from build123d import *

# Parameters (mm, degrees)
SKETCH1_W           = 44.45
SKETCH1_H           = 44.45
BOSS_EXTRUDE1_DEPTH = 6.35
SKETCH2_W           = 31.75
SKETCH2_H           = 31.75
BOSS_EXTRUDE2_DEPTH = 25.4
SKETCH3_W           = 44.45
SKETCH3_H           = 44.45
BOSS_EXTRUDE3_DEPTH = 6.35
SKETCH4_W           = 25.4
SKETCH4_H           = 25.4
CUT_EXTRUDE1_DEPTH  = 39.1
CUT_EXTRUDE3_START  = -7.35
SKETCH6_R           = 2.413
CUT_EXTRUDE3_DEPTH  = 40.1
CIRPATTERN1_COUNT   = 4


with BuildPart() as part:
    # Sketch1 → Boss-Extrude1 (new body)
    with BuildSketch(Plane(origin=(0, 0, 0), x_dir=(1, 0, 0), z_dir=(0, 1, 0))):
        Rectangle(SKETCH1_W, SKETCH1_H)
    extrude(amount=BOSS_EXTRUDE1_DEPTH)

    # Sketch2 → Boss-Extrude2 (add)
    with BuildSketch(Plane(origin=(0, 6.35, 0), x_dir=(1, 0, 0), z_dir=(0, 1, 0))):
        Rectangle(SKETCH2_W, SKETCH2_H)
    extrude(amount=BOSS_EXTRUDE2_DEPTH)

    # Sketch3 → Boss-Extrude3 (add)
    with BuildSketch(Plane(origin=(0, 31.75, 0), x_dir=(1, 0, 0), z_dir=(0, 1, 0))):
        Rectangle(SKETCH3_W, SKETCH3_H)
    extrude(amount=BOSS_EXTRUDE3_DEPTH)

    # Sketch4 → Cut-Extrude1 (cut, through all)
    with BuildSketch(Plane(origin=(0, 38.1, 0), x_dir=(1, 0, 0), z_dir=(0, 1, 0))):
        Rectangle(SKETCH4_W, SKETCH4_H)
    extrude(amount=-CUT_EXTRUDE1_DEPTH, mode=Mode.SUBTRACT)

    # Sketch6 → Cut-Extrude3 (cut)
    with BuildSketch(Plane.XZ.offset(-31.75).offset(CUT_EXTRUDE3_START)):
        with Locations((19.05, 19.05)):
            Circle(SKETCH6_R)
    cut_extrude3 = extrude(amount=CUT_EXTRUDE3_DEPTH, mode=Mode.SUBTRACT)

    # CirPattern1: Cut-Extrude3 ×4 about axis
    cirpattern1_axis = Axis((0, 0, 0), (0, 1, 0))
    for i in range(1, CIRPATTERN1_COUNT):
        add(cut_extrude3.rotate(cirpattern1_axis, i * 360 / CIRPATTERN1_COUNT), mode=Mode.SUBTRACT)


solid = part.part
For this review, take the finished solid that the model builds, in its own axes (mm). A direction names the side the tool comes from. Round coordinates to 2 decimals unless told otherwise and drop trailing zeros. Loops run counter-clockwise (first coordinate to the right, second up) from the corner with the lowest first, then second, coordinate; pieces in that order, holes last. Notation, with made-up numbers: (44.25, 25.25) - (78.25, 25.25) arc R32 ccw to (78.25, 64.25) - close; hole circle Ø4 at (-32, -28). An arc over 180 degrees is marked (long way). Answer as CSV lines item,"result".
(1) Insertion check: P1, Ø1.5, axis at x = -3.5, y = 22, coming from the +Z side (3 decimals); P2, Ø20.5, axis at y = 21, z = 6, coming from the -X side (3 decimals); P3, Ø12, axis at y = 15.5, z = -10, coming from the +X side (3 decimals). Each pin has a flat end and moves straight along its axis. Give the tip position at first contact, or say it passes through.
Checked values:
P1,"stops at z = 15.875"
P2,"stops at x = -15.875"
P3,"stops at x = 15.875"
(2) Consider section D-D on y = 24.5. Give the boundary of the cut face in (x, z) (3 decimals), then the cut area to 3 significant figures.
Checked values:
outline,"(-15.875, -15.875) - (15.875, -15.875) - (15.875, 15.875) - (-15.875, 15.875) - close; hole (-12.7, -12.7) - (12.7, -12.7) - (12.7, 12.7) - (-12.7, 12.7) - close"
area,"363 mm2"
(3) Tool access review of faces 5 (the face through (-17, 31.75, -2)), 6 (the face through (-12.7, 19, 0)), 7 (the face through (-15.875, 19, 0)), 8 (the face through (0, 3, -22.225)): name each direction out of +Z, -Z, +X, -X, +Y, -Y from which nothing blocks a thin tool from reaching the whole face with its end or side.
Checked values:
face 5,"none"
face 6,"+Y, -Y"
face 7,"+Z, -Z, -X"
face 8,"-Z, +X, -X, +Y, -Y"
(4) Consider section B-B on y = 3. Give the boundary of the cut face in (x, z) (3 decimals), then the cut area to 3 significant figures.
Checked values:
outline,"(-22.225, -22.225) - (22.225, -22.225) - (22.225, 22.225) - (-22.225, 22.225) - close; hole circle Ø4.826 at (-19.05, -19.05); hole circle Ø4.826 at (-19.05, 19.05); hole (-12.7, -12.7) - (12.7, -12.7) - (12.7, 12.7) - (-12.7, 12.7) - close; hole circle Ø4.826 at (19.05, -19.05); hole circle Ø4.826 at (19.05, 19.05)"
area,"1,260 mm2"
(5) Consider section A-A on z = 2.5. Give the boundary of the cut face in (x, y) (3 decimals).
Checked values:
outline,"(-22.225, 0) - (-12.7, 0) - (-12.7, 38.1) - (-22.225, 38.1) - (-22.225, 31.75) - (-15.875, 31.75) - (-15.875, 6.35) - (-22.225, 6.35) - close; (12.7, 0) - (22.225, 0) - (22.225, 6.35) - (15.875, 6.35) - (15.875, 31.75) - (22.225, 31.75) - (22.225, 38.1) - (12.7, 38.1) - close"
(6) Wall thickness on line 1 (X direction, y = 34.5, z = 19.05) (3 decimals); line 2 (Z direction, x = 0.5, y = 25.5) (3 decimals): over which ranges is each line inside the solid? List them lowest first.
Checked values:
line 1,"x = -22.225 to -21.463, -16.637 to 16.637, 21.463 to 22.225"
line 2,"z = -15.875 to -12.7, 12.7 to 15.875"
(7) Mouldability with a two-part tool opening along X and no side actions: class faces 1 (the face through (-22.225, 3, 0)), 2 (the face through (-21.442, 34.969, 18.736)), 3 (the face through (22.225, 3, 0)), 4 (the face through (0, 35, 22.225)) as +X half, -X half, draft (parallel to the pull), parting line (faces both ways), or undercut.
Checked values:
face 1,"-X half"
face 2,"undercut"
face 3,"+X half"
face 4,"draft"
(8) Consider section C-C on x = 19.05. Give the boundary of the cut face in (y, z) (3 decimals), then the cut area to 3 significant figures.
Checked values:
outline,"(0, -22.225) - (6.35, -22.225) - (6.35, -21.463) - (0, -21.463) - close; (0, -16.637) - (6.35, -16.637) - (6.35, 16.637) - (0, 16.637) - close; (0, 21.463) - (6.35, 21.463) - (6.35, 22.225) - (0, 22.225) - close; (31.75, -22.225) - (38.1, -22.225) - (38.1, -21.463) - (31.75, -21.463) - close; (31.75, -16.637) - (38.1, -16.637) - (38.1, 16.637) - (31.75, 16.637) - close; (31.75, 21.463) - (38.1, 21.463) - (38.1, 22.225) - (31.75, 22.225) - close"
area,"442 mm2"
